Part print with two shaded views. Sizes in mm from the minimum x, y, z corner. A direction names the side the tool comes from. Round coordinates to 2 decimals unless told otherwise and drop trailing zeros. Order: outer loops, then holes, each group sorted by start corner. A loop starts at its lowest first (then second) coordinate and runs counter-clockwise, first axis right, second up. Notation, with made-up numbers: M -35.75,15 L -26.75,15 A29 cw -26.75,53 Z; hole C 57.5,-11.5 d8. An arc over 180 degrees is marked long. One line per question, with ' | ' between items. Start each with the question number.
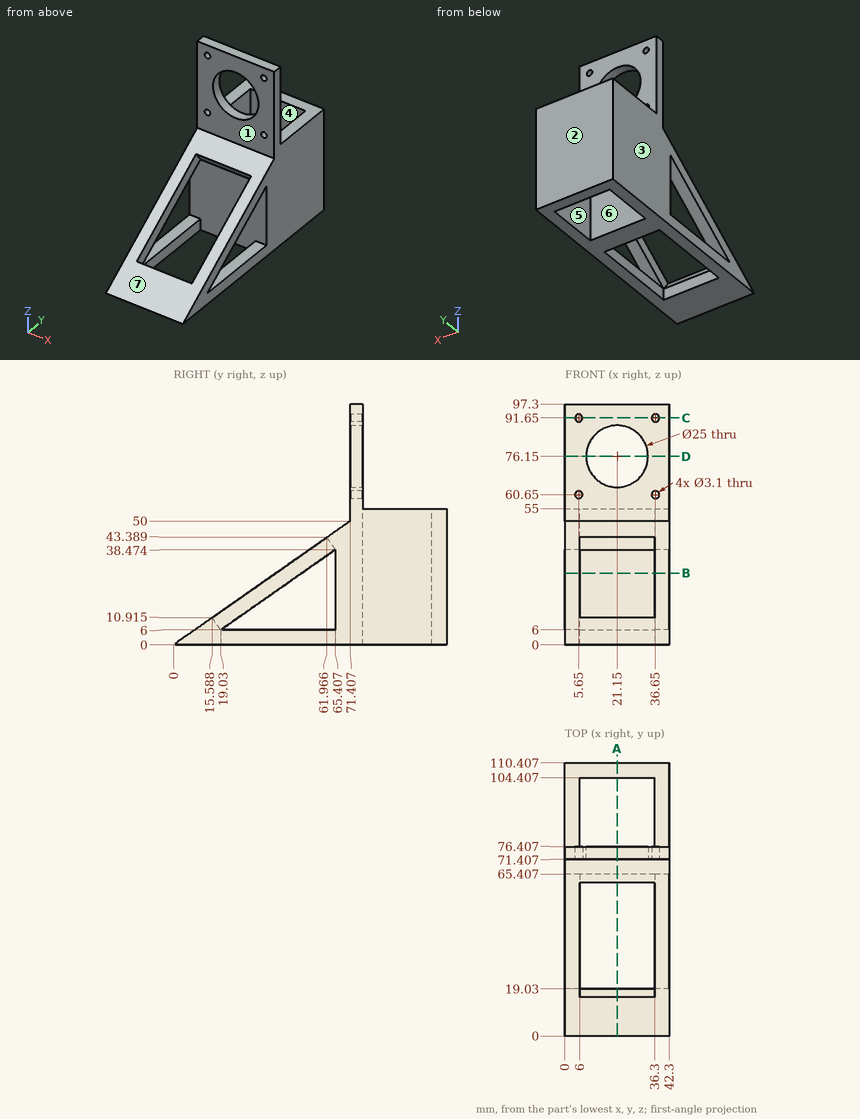
Item 1: Wall check: line 1 along Z through (x, y) = (36.65, 73.3); line 2 along X through (y, z) = (81.5, 40.5); line 3 along Z through (x, y) = (21, 74). Give the ranges that are in metal, low to high. Write a range as [from, to].
Item 2: Cut at B-B on z = 29. Write the cut outline in (x, y).
Item 3: Cut at D-D on z = 76.15. Write the cut outline in (x, y), then the cut area to 3 significant figures.
Item 4: Two-plate mould, pull along Y, no slides. Class the marked faces 1, 2, 3 and 4: +Y half, -Y half, draft (parallel to the pull), parting line (faces both ways), or undercut.
Item 5: Flat gauge pins, fed straight in: pin 1 (3.5 mm diameter, centred on x = 36.65, z = 91.65, fed in from +Y); pin 2 (6.5 mm diameter, centred on y = 47, z = 3.5, fed in from -X); pin 3 (1 mm diameter, centred on x = 4.5, z = 66, fed in from -Y); pin 4 (5 mm diameter, centred on x = 3, y = 46.5, fed in from +Z). Where does each tip first touch, or does it go through?
Item 6: Tool access for the marked faces 5, 6 and 7: list every direction of +Z, -Z, +X, -X, +Y, -Y with a clear straight run to the whole face (end or side of a thin tool).
Item 7: Cut at A-A on x = 21.15. Count the separate pieces of the cut face and the enclosed holes in it, then the cut area to 3 significant figures.
Item 8: Cut at C-C on z = 91.65. Write the cut outline in (x, y).
Results found:
1) line 1: z = [0, 59.1], [62.2, 90.1], [93.2, 97.3] | line 2: x = [0, 6], [36.3, 42.3] | line 3: z = [0, 63.65], [88.65, 97.3]
2) outline: M 0,41.42 L 6,41.42 L 6,51.88 L 0,51.88 Z; M 0,65.41 L 42.3,65.41 L 42.3,110.41 L 0,110.41 Z; M 36.3,41.42 L 42.3,41.42 L 42.3,51.88 L 36.3,51.88 Z; hole M 6,76.41 L 36.3,76.41 L 36.3,104.41 L 6,104.41 Z
3) outline: M 0,71.41 L 8.65,71.41 L 8.65,76.41 L 0,76.41 Z; M 33.65,71.41 L 42.3,71.41 L 42.3,76.41 L 33.65,76.41 Z | area: 86.5 mm^2
4) face 1: -Y half | face 2: +Y half | face 3: draft | face 4: undercut
5) pin 1: stops at y = 76.41 | pin 2: stops at x = 0 | pin 3: stops at y = 71.41 | pin 4: stops at z = 34.31
6) face 5: +Z, -Z | face 6: +Z | face 7: +Z, +X, -X, -Y
7) separate pieces: 4 | enclosed holes: 0 | area: 1,110 mm^2
8) outline: M 0,71.41 L 4.1,71.41 L 4.1,76.41 L 0,76.41 Z; M 7.2,71.41 L 35.1,71.41 L 35.1,76.41 L 7.2,76.41 Z; M 38.2,71.41 L 42.3,71.41 L 42.3,76.41 L 38.2,76.41 Z
